```python
from build123d import *

# Parameters (mm, degrees)
BOSS_EXTRUDE1_DEPTH = 4
SKETCH2_R           = 2
CUT_EXTRUDE1_DEPTH  = 10
SKETCH3_R           = 30
CUT_EXTRUDE2_DEPTH  = 10
SKETCH4_R           = 40.429464175
CUT_EXTRUDE3_DEPTH  = 69.109947193
FILLET5_R           = 2
FILLET6_R           = 2


with BuildPart() as part:
    # Sketch1 → Boss-Extrude1 (new body)
    with BuildSketch(Plane.XY):
        Polygon((-46.844369636, 32.999996521), (-41.844369636, 32.999996711), (-41.844366793, 42.000003289), (-31.344369977, 41.999997109), (-31.344370091, 44.999997109), (-24.344370091, 44.999997374), (-24.344370205, 47.999997374), (25.655629795, 47.99999927), (25.655629909, 44.99999927), (32.655629909, 44.999999535), (32.655630023, 41.999999535), (43.155633207, 42.000000067), (43.155630364, 32.999999933), (48.155630364, 33.000000123), (48.155632866, -32.999999877), (43.155630364, -32.999999933), (43.155633207, -42.000000067), (32.655630023, -41.999999535), (32.655629909, -44.999999535), (25.655629909, -44.99999927), (25.655629795, -47.99999927), (-24.344370205, -47.999997374), (-24.344370091, -44.999997374), (-31.344370091, -44.999997109), (-31.344369977, -41.999997109), (-41.844366793, -42.000003289), (-41.844369636, -32.999996711), (-46.844369636, -32.999996521), align=None)
    extrude(amount=BOSS_EXTRUDE1_DEPTH)

    # Sketch2 → Cut-Extrude1 (cut)
    with BuildSketch(Plane.XY.offset(4)):
        with Locations((-36.344424402, 38.000040227)):
            Circle(SKETCH2_R)
        with Locations((37.655687631, -38.000043584)):
            Circle(SKETCH2_R)
        with Locations((37.655603638, 37.999999725)):
            Circle(SKETCH2_R)
        with Locations((-36.344340408, -38.000003081)):
            Circle(SKETCH2_R)
    extrude(amount=-CUT_EXTRUDE1_DEPTH, mode=Mode.SUBTRACT)

    # Sketch3 → Cut-Extrude2 (cut)
    with BuildSketch(Plane.XY.offset(4)):
        Circle(SKETCH3_R)
    extrude(amount=-CUT_EXTRUDE2_DEPTH, mode=Mode.SUBTRACT)

    # Sketch4 → Cut-Extrude3 (cut, through all)
    with BuildSketch(Plane.XY.offset(4)):
        Circle(SKETCH4_R)
    extrude(amount=-CUT_EXTRUDE3_DEPTH, mode=Mode.SUBTRACT)

    # Fillet5
    fillet5_edges = [part.edges().sort_by_distance(p)[0] for p in [
        (-40.429464175, 0, 4),
    ]]
    fillet(fillet5_edges, radius=FILLET5_R)

    # Fillet6
    fillet6_edges = [part.edges().sort_by_distance(p)[0] for p in [
        (-40.429464175, 0, 0),
    ]]
    fillet(fillet6_edges, radius=FILLET6_R - 0.0001)  # a hair under: the kernel refuses the full size


solid = part.part
```
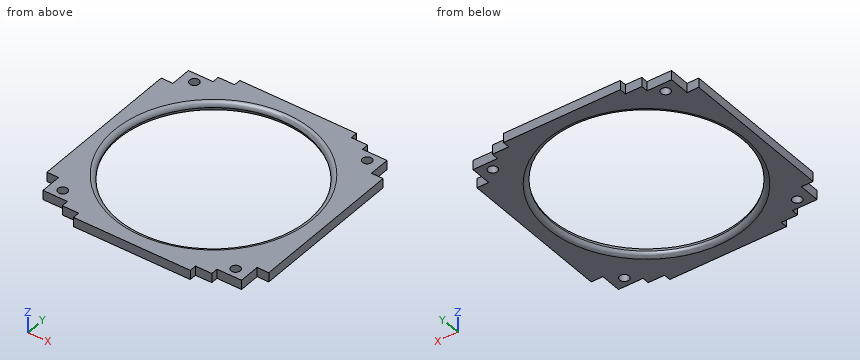
Verification items for the finished model (mm, model axes). Give positions to 0.01 mm unless a question says otherwise; leave off trailing zeros. Put each result on its own line as item: value.
Q1. Section check C-C on z = 1.1. Count the separate pieces of the cut face and the enclosed holes in it, and give its area (3 significant figures).
Result:
separate pieces: 1
enclosed holes: 5
area: 3,240 mm2
Q2. Scan lines: probe 1 along Y at (x, z) = (-28, 1.6); probe 2 along Y at (x, z) = (-8, 1.7); probe 3 along X at (y, z) = (-11, 2.1). Record each from-to range of solid material in increasing order. Write a range as from..to.
Result:
probe 1: -45..-29.22, 29.22..45
probe 2: -48..-39.65, 39.65..48
probe 3: -46.84..-38.91, 38.91..48.16
Q3. Depth check by flat-ended pin: P1, Ø2, axis at x = 30.5, z = 2, coming from the +Y side; P2, Ø1.2, axis at x = 45.5, z = 1.5, coming from the -Y side; P3, Ø2, axis at y = -39, z = 2.5, coming from the +X side. Enter the tip coordinate at first touch or a pass-through.
Result:
P1: y = 45
P2: y = -33
P3: x = 43.16
